Geometry check sheet. Reference: the model listing, model coordinates, mm. A direction names the side the tool comes from. Coordinates: 2 decimals unless noted, no trailing zeros. Write each loop counter-clockwise with the first axis right and the second up, starting at its lowest first coordinate (ties: lowest second). Pieces come first, ordered by that corner, then holes. Notation, with made-up numbers: (21, 57) -> (32, 57) arc R29 ccw to (32, 78) -> close; hole circle Ø3 at (3, 63.25). An arc over 180 degrees is marked (long way). Use a Markdown table: item, result.
```python
from build123d import *

# Parameters (mm, degrees)
SKETCH_1_W          = 10
SKETCH_1_H          = 20
SKETCH_1_W_2        = 7
SKETCH_1_H_2        = 17
EXTRUDE_1_DEPTH     = 525
SKETCH_2_R          = 2.15
SKETCH_2_R_2        = 2.5
CUT_EXTRUDE_1_DEPTH = 526.19044165
CUT_EXTRUDE_2_REACH = 527.405
SKETCH_3_R          = 2.15


with BuildPart() as part:
    # ｽｹｯﾁ1 → 押し出し-薄板1 (new body)
    with BuildSketch(Plane(origin=(0, 0, 0), x_dir=(0, 0, -1), z_dir=(1, 0, 0))):
        Rectangle(SKETCH_1_W, SKETCH_1_H)
        Rectangle(SKETCH_1_W_2, SKETCH_1_H_2, mode=Mode.SUBTRACT)
    extrude(amount=EXTRUDE_1_DEPTH)

    # ｽｹｯﾁ2 → ｶｯﾄ - 押し出し1 (cut, through all)
    with BuildSketch(Plane.XY.offset(5)):
        with Locations((282.5, 0)):
            Circle(SKETCH_2_R)
        with Locations((262.5, 0)):
            Circle(SKETCH_2_R)
        with Locations(Location((242.5, 0, 0), (0, 0, 90))):
            Circle(SKETCH_2_R)
        with Locations((487.5, 0)):
            Circle(SKETCH_2_R_2)
        with Locations(Location((37.5, 0, 0), (0, 0, 90))):
            Circle(SKETCH_2_R_2)
        with Locations((520, 5)):
            Circle(SKETCH_2_R)
        with Locations(Location((520, -5, 0), (0, 0, 90))):
            Circle(SKETCH_2_R)
        with Locations((500, 5)):
            Circle(SKETCH_2_R)
        with Locations(Location((500, -5, 0), (0, 0, 90))):
            Circle(SKETCH_2_R)
        with Locations((25, -5)):
            Circle(SKETCH_2_R)
        with Locations(Location((25, 5, 0), (0, 0, 90))):
            Circle(SKETCH_2_R)
        with Locations((5, -5)):
            Circle(SKETCH_2_R)
        with Locations(Location((5, 5, 0), (0, 0, 90))):
            Circle(SKETCH_2_R)
    extrude(amount=-CUT_EXTRUDE_1_DEPTH, mode=Mode.SUBTRACT)

    # ｶｯﾄ - 押し出し2: up to this face of the body (flat: up to its plane)
    cut_extrude_2_end = Plane(part.part.faces().sort_by_distance((262.5, -10, 0))[0])
    # ｽｹｯﾁ3 → ｶｯﾄ - 押し出し2 (cut, up to the picked face)
    with BuildSketch(Plane(origin=(0, 10, 0), x_dir=(1, 0, 0), z_dir=(0, 1, 0)), mode=Mode.PRIVATE) as cut_extrude_2_sk1:
        with Locations(Location((5, 0, 0), (0, 0, 270))):
            Circle(SKETCH_3_R)
    cut_extrude_2_tool1 = split(extrude(cut_extrude_2_sk1.sketch, amount=-CUT_EXTRUDE_2_REACH, mode=Mode.PRIVATE), bisect_by=cut_extrude_2_end, keep=Keep.BOTH, mode=Mode.PRIVATE)
    # ｽｹｯﾁ3 → ｶｯﾄ - 押し出し2 (cut, up to the picked face)
    with BuildSketch(Plane(origin=(0, 10, 0), x_dir=(1, 0, 0), z_dir=(0, 1, 0)), mode=Mode.PRIVATE) as cut_extrude_2_sk2:
        with Locations(Location((25, 0, 0), (0, 0, 270))):
            Circle(SKETCH_3_R)
    cut_extrude_2_tool2 = split(extrude(cut_extrude_2_sk2.sketch, amount=-CUT_EXTRUDE_2_REACH, mode=Mode.PRIVATE), bisect_by=cut_extrude_2_end, keep=Keep.BOTH, mode=Mode.PRIVATE)
    # ｽｹｯﾁ3 → ｶｯﾄ - 押し出し2 (cut, up to the picked face)
    with BuildSketch(Plane(origin=(0, 10, 0), x_dir=(1, 0, 0), z_dir=(0, 1, 0)), mode=Mode.PRIVATE) as cut_extrude_2_sk3:
        with Locations(Location((500, 0, 0), (0, 0, 270))):
            Circle(SKETCH_3_R)
    cut_extrude_2_tool3 = split(extrude(cut_extrude_2_sk3.sketch, amount=-CUT_EXTRUDE_2_REACH, mode=Mode.PRIVATE), bisect_by=cut_extrude_2_end, keep=Keep.BOTH, mode=Mode.PRIVATE)
    # ｽｹｯﾁ3 → ｶｯﾄ - 押し出し2 (cut, up to the picked face)
    with BuildSketch(Plane(origin=(0, 10, 0), x_dir=(1, 0, 0), z_dir=(0, 1, 0)), mode=Mode.PRIVATE) as cut_extrude_2_sk4:
        with Locations(Location((520, 0, 0), (0, 0, 270))):
            Circle(SKETCH_3_R)
    cut_extrude_2_tool4 = split(extrude(cut_extrude_2_sk4.sketch, amount=-CUT_EXTRUDE_2_REACH, mode=Mode.PRIVATE), bisect_by=cut_extrude_2_end, keep=Keep.BOTH, mode=Mode.PRIVATE)
    add(cut_extrude_2_tool1.solids().sort_by(Axis((5, 10, 0), (0, -1, 0)))[0], mode=Mode.SUBTRACT)
    add(cut_extrude_2_tool2.solids().sort_by(Axis((25, 10, 0), (0, -1, 0)))[0], mode=Mode.SUBTRACT)
    add(cut_extrude_2_tool3.solids().sort_by(Axis((500, 10, 0), (0, -1, 0)))[0], mode=Mode.SUBTRACT)
    add(cut_extrude_2_tool4.solids().sort_by(Axis((520, 10, 0), (0, -1, 0)))[0], mode=Mode.SUBTRACT)


solid = part.part
```
Item 1: Thickness scan on L1, parallel to X at y = -9, z = 0; L2, parallel to Z at x = 472, y = -1; L3, parallel to Y at x = 25, z = 3.9. Record the ranges inside material, lowest first. Write a range as [from, to].
Answer block:
| item | result |
|---|---|
| L1 | x = [0, 2.85], [7.15, 22.85], [27.15, 497.85], [502.15, 517.85], [522.15, 525] |
| L2 | z = [-5, -3.5], [3.5, 5] |
| L3 | y = [-10, -7.15], [-2.85, 2.85], [7.15, 10] |
Item 2: Tool access check on faces 1 (the flat face through (259, 0, -3.5)), 2 (the flat face through (259, 0, -5)). Record the directions out of +Z, -Z, +X, -X, +Y, -Y that give a thin tool (end or side, any length) a straight path to the whole face; none if there is none.
Answer block:
| item | result |
|---|---|
| face 1 | +X, -X |
| face 2 | -Z, +X, -X, +Y, -Y |
Item 3: Mould release check, pull along Y, two halves, no side actions. Record for faces 3 (the flat face through (259, -10, 0)), 4 (the flat face through (259, 10, 0)), 5 (the flat face through (525, 0.1, 4.5)), 6 (the flat face through (259, 0, 3.5)): +Y half, -Y half, draft (parallel to the pull), parting line (faces both ways), or undercut.
Answer block:
| item | result |
|---|---|
| face 3 | -Y half |
| face 4 | +Y half |
| face 5 | draft |
| face 6 | undercut |
Item 4: Section check A-A on x = 453. Record the boundary of the cut face in (y, z).
Answer block:
| item | result |
|---|---|
| outline | (-10, -5) -> (10, -5) -> (10, 5) -> (-10, 5) -> close; hole (-8.5, -3.5) -> (8.5, -3.5) -> (8.5, 3.5) -> (-8.5, 3.5) -> close |
